The drawing under review shows one solid part. Ordinate dimensions are in mm from its lowest x, y, z. Round coordinates to 2 decimals unless told otherwise and drop trailing zeros. Order: outer loops, then holes, each group sorted by start corner. A loop starts at its lowest first (then second) coordinate and runs counter-clockwise, first axis right, second up. Notation, with made-up numbers: (22, 74.5) - (55, 74.5) arc R23 ccw to (55, 105.5) - close; hole circle Ø3 at (-34, 43.5). An arc over 180 degrees is marked (long way). One line per question, with ' | ' between items.
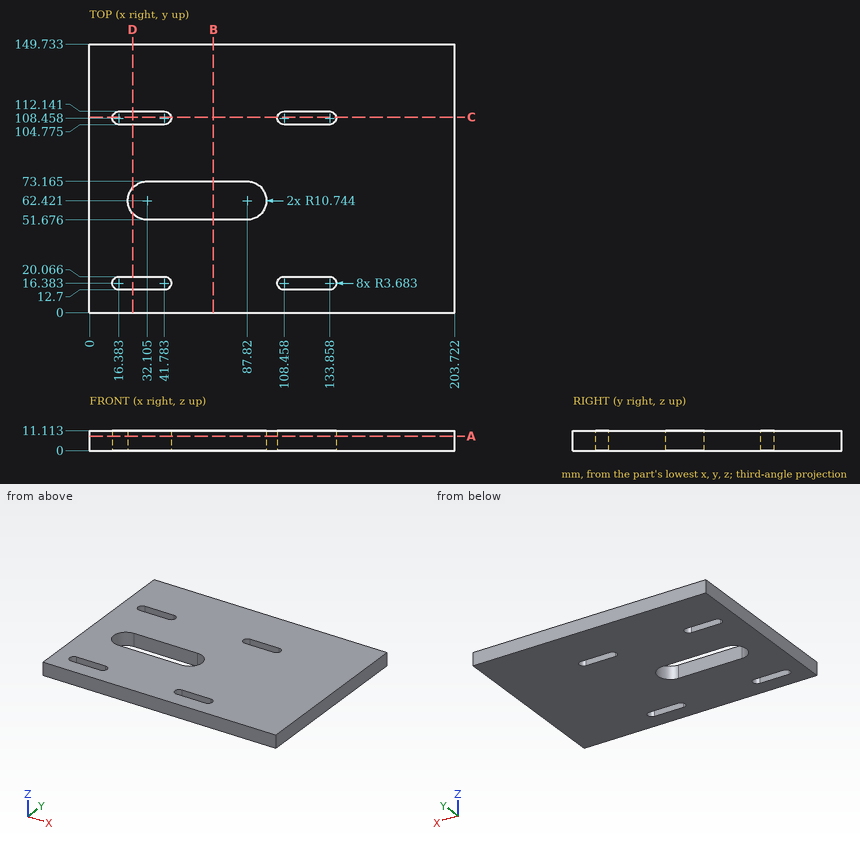
(1) We need section D-D on x = 24. State the section outline as (y, z) points (1 decimal), plus the area to 3 significant figures.
Output values:
outline: (0, 0) - (12.7, 0) - (12.7, 11.1) - (0, 11.1) - close; (20.1, 0) - (55.4, 0) - (55.4, 11.1) - (20.1, 11.1) - close; (69.5, 0) - (104.8, 0) - (104.8, 11.1) - (69.5, 11.1) - close; (112.1, 0) - (149.7, 0) - (149.7, 11.1) - (112.1, 11.1) - close | area: 1,340 mm^2
(2) We need section B-B on x = 69. State the section outline as (y, z) points (1 decimal).
Output values:
outline: (0, 0) - (51.7, 0) - (51.7, 11.1) - (0, 11.1) - close; (73.2, 0) - (149.7, 0) - (149.7, 11.1) - (73.2, 11.1) - close
(3) Insertion check: pin 1 (6 mm diameter, centred on x = 41.5, z = 6.5, fed in from -Y). The pin has a flat end and moves straight along its axis. Give the tip position at first contact, or say it passes through.
Output values:
pin 1: y = 0
(4) For probe 1 along X at (y, z) = (109, 4.25) (1 decimal); probe 2 along Y at (x, z) = (38.5, 5.75) (1 decimal); probe 3 along Y at (x, z) = (68, 2.5) (1 decimal), list the stretches that pass through material, from the lowest coordinate up. Write a range as [from, to].
Output values:
probe 1: [0, 12.7], [45.4, 104.8], [137.5, 203.7] | probe 2: [0, 12.7], [20.1, 51.7], [73.2, 104.8], [112.1, 149.7] | probe 3: [0, 51.7], [73.2, 149.7]
(5) We need section C-C on y = 109. State the section outline as (x, z) points (1 decimal), plus the area to 3 significant figures.
Output values:
outline: (0, 0) - (12.7, 0) - (12.7, 11.1) - (0, 11.1) - close; (45.4, 0) - (104.8, 0) - (104.8, 11.1) - (45.4, 11.1) - close; (137.5, 0) - (203.7, 0) - (203.7, 11.1) - (137.5, 11.1) - close | area: 1,540 mm^2
(6) We need section A-A on z = 8. State the section outline as (x, y) points (1 decimal), plus the area to 3 significant figures.
Output values:
outline: (0, 0) - (203.7, 0) - (203.7, 149.7) - (0, 149.7) - close; hole (16.4, 12.7) - (41.8, 12.7) arc R3.7 ccw to (41.8, 20.1) - (16.4, 20.1) arc R3.7 ccw to start; hole (16.4, 104.8) - (41.8, 104.8) arc R3.7 ccw to (41.8, 112.1) - (16.4, 112.1) arc R3.7 ccw to start; hole (32.1, 51.7) - (87.8, 51.7) arc R10.7 ccw to (87.8, 73.2) - (32.1, 73.2) arc R10.7 ccw to start; hole (108.5, 12.7) - (133.9, 12.7) arc R3.7 ccw to (133.9, 20.1) - (108.5, 20.1) arc R3.7 ccw to start; hole (108.5, 104.8) - (133.9, 104.8) arc R3.7 ccw to (133.9, 112.1) - (108.5, 112.1) arc R3.7 ccw to start | area: 28,000 mm^2
